```python
from build123d import *

# Parameters (mm, degrees)
FILLET_1_R          = 0.2
CHAMFER_1_SIZE      = 0.2
CUT_EXTRUDE_1_DEPTH = 1.5


with BuildPart() as part:
    # 草图2 → 旋转1 (revolve)
    with BuildSketch(Plane(origin=(0, 0, 0), x_dir=(0, 0, -1), z_dir=(1, 0, 0))):
        Polygon((0, 0), (0, 2.3), (2.5, 2.3), (2.5, 1.25), (7.5, 1.25), (7.5, 0), align=None)
    revolve(axis=Axis((0, 0, -7.5), (0, 0, 1)))

    # 圆角1
    fillet_1_edges = [part.edges().sort_by_distance(p)[0] for p in [
        (0, -2.3, -2.5),
        (0, -2.3, 0),
    ]]
    fillet(fillet_1_edges, radius=FILLET_1_R)

    # 倒角1
    chamfer_1_edges = [part.edges().sort_by_distance(p)[0] for p in [
        (0, -1.25, -7.5),
    ]]
    chamfer(chamfer_1_edges, length=CHAMFER_1_SIZE)

    # 草图3 → 切除-拉伸1 (cut)
    with BuildSketch(Plane.XY):
        Polygon((1.154700538, 0), (0.577350269, 1), (-0.577350269, 1), (-1.154700538, 0), (-0.577350269, -1), (0.577350269, -1), align=None)
    extrude(amount=-CUT_EXTRUDE_1_DEPTH, mode=Mode.SUBTRACT)


solid = part.part
```
Work out the finished part from the listing and answer in its coordinate system (mm). A direction names the side the tool comes from. Round coordinates to 2 decimals unless told otherwise and drop trailing zeros. Write each loop counter-clockwise with the first axis right and the second up, starting at its lowest first coordinate (ties: lowest second). Pieces come first, ordered by that corner, then holes.
1) Which of the six approach directions +Z, -Z, +X, -X, +Y, -Y give full straight-line access (tool end or side, diameter ignored) to faces 4 (the face through (1.22, -0.27, -4.93)), 5 (the face through (0, -1, -1)), 6 (the face through (1, -1, 0))?
2) Flat-ended cylindrical pins translate along their axes: P1, Ø1.6, axis at x = 0, y = 0, coming from the +Z side; P2, Ø1.5, axis at x = 1, z = -4.5, coming from the +Y side. Find the tip coordinate at first contact, or state that the pin passes through.
3) Determine the mould class of faces 1 (the face through (0, 1, -1)), 2 (the face through (1.4, -1.825, -1.265)), 3 (the face through (1, 1, -2.5)) for opening direction Y: pulls with the +Y half, pulls with the -Y half, needs draft (parallel to the pull), parting line crosses it, or undercut.
4) A cutting plane is placed at C-C on z = -3.25. Determine the outline of the cut face in (x, y).
5) A cutting plane is placed at B-B on x = 0. Determine the outline of the cut face in (y, z), and give its area (3 significant figures).
6) A cutting plane is placed at A-A on z = -1. Determine the outline of the cut face in (x, y).
7) Consider probe 1 along Z at (x, y) = (-1.75, 0.45); probe 2 along Z at (x, y) = (0.25, -0.1); probe 3 along Y at (x, z) = (0.4, -0.5). Determine where each line is inside the solid, lowest interval first.
Entries:
1. face 4: -Z
1. face 5: +Z
1. face 6: +Z, +X, -X, +Y, -Y
2. P1: stops at z = -1.5
2. P2: stops at y = 1.22
3. face 1: undercut
3. face 2: parting line crosses it
3. face 3: needs draft
4. outline: circle Ø2.5 at (0, 0)
5. outline: (-2.3, -2.3) arc R0.2 ccw to (-2.1, -2.5) - (-1.25, -2.5) - (-1.25, -7.3) - (-1.05, -7.5) - (1.05, -7.5) - (1.25, -7.3) - (1.25, -2.5) - (2.1, -2.5) arc R0.2 ccw to (2.3, -2.3) - (2.3, -0.2) arc R0.2 ccw to (2.1, 0) - (1, 0) - (1, -1.5) - (-1, -1.5) - (-1, 0) - (-2.1, 0) arc R0.2 ccw to (-2.3, -0.2) - close
5. area: 20.9 mm2
6. outline: circle Ø4.6 at (0, 0); hole (-1.15, 0) - (-0.58, -1) - (0.58, -1) - (1.15, 0) - (0.58, 1) - (-0.58, 1) - close
7. probe 1: z = -2.5 to 0
7. probe 2: z = -7.5 to -1.5
7. probe 3: y = -2.26 to -1, 1 to 2.26
